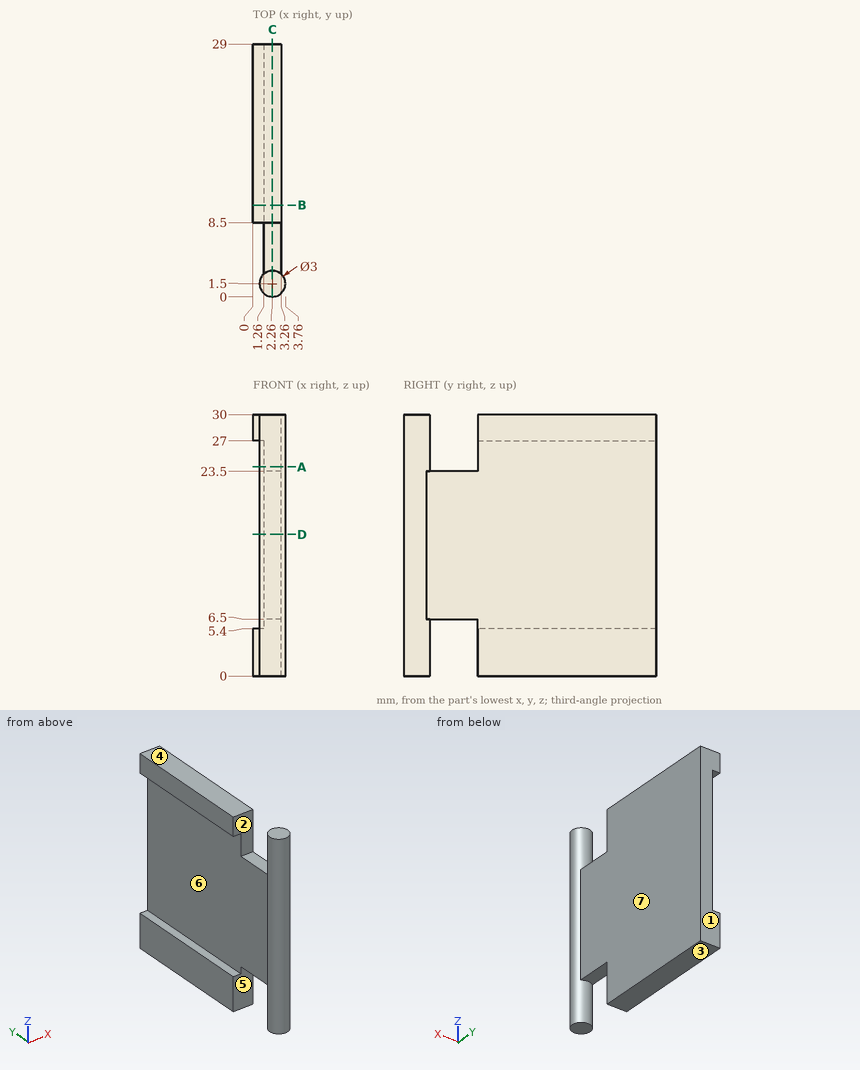
Check sheet for the drawn part. Datum: minimum x, y, z corner. Units: mm. A direction names the side the tool comes from. Round coordinates to 2 decimals unless told otherwise and drop trailing zeros. Order: outer loops, then holes, each group sorted by start corner. A loop starts at its lowest first (then second) coordinate and runs counter-clockwise, first axis right, second up. Notation, with made-up numbers: (25.5, 72.25) -> (70.5, 72.25) arc R26 ccw to (70.5, 103.25) -> close; hole circle Ø7 at (-24, -5). An arc over 180 degrees is marked (long way). Use CSV: the item, a comma, the result in double quotes.
(1) Cross-section at D-D (z = 16.25). Record the boundary of the cut face in (x, y).
Worked out:
outline,"(1.26, 2.62) arc R1.5 ccw (long way) to (3.26, 2.62) -> (3.26, 29) -> (1.26, 29) -> close"
(2) Draft check along Y on the marked faces 1, 2 and 3. Enter one of: pulls with the +Y half, pulls with the -Y half, needs draft (parallel to the pull), parting line crosses it, or undercut.
Worked out:
face 1,"pulls with the +Y half"
face 2,"undercut"
face 3,"needs draft"
(3) Cross-section at A-A (z = 24). Record the boundary of the cut face in (x, y), and give its area (3 significant figures).
Worked out:
outline,"circle Ø3 at (2.26, 1.5); (1.26, 8.5) -> (3.26, 8.5) -> (3.26, 29) -> (1.26, 29) -> close"
area,"48.1 mm²"
(4) Tool access check on the marked faces 4, 5, 6 and 7. Record the directions out of +Z, -Z, +X, -X, +Y, -Y that give a thin tool (end or side, any length) a straight path to the whole face; none if there is none.
Worked out:
face 4,"+Z, +X, -X, +Y, -Y"
face 5,"-Z, +X, -X"
face 6,"-X, +Y"
face 7,"+Z, -Z, +X, +Y"
(5) Cross-section at C-C (x = 2.26). Record the boundary of the cut face in (y, z).
Worked out:
outline,"(0, 0) -> (3, 0) -> (3, 6.5) -> (8.5, 6.5) -> (8.5, 0) -> (29, 0) -> (29, 30) -> (8.5, 30) -> (8.5, 23.5) -> (3, 23.5) -> (3, 30) -> (0, 30) -> close"
(6) Cross-section at B-B (y = 10.5). Record the boundary of the cut face in (x, z).
Worked out:
outline,"(0, 0) -> (3.26, 0) -> (3.26, 30) -> (0, 30) -> (0, 27) -> (1.26, 27) -> (1.26, 5.4) -> (0, 5.4) -> close"
(7) Depth check by flat-ended pin: pin 1 (0.6 mm diameter, centred on x = 2.5, y = 5.5, fed in from -Z); pin 2 (11 mm diameter, centred on y = 19.5, z = 16.5, fed in from -X); pin 3 (13 mm diameter, centred on y = 13.5, z = 11.5, fed in from +X). Enter the tip coordinate at first touch or a pass-through.
Worked out:
pin 1,"z = 6.5"
pin 2,"x = 1.26"
pin 3,"x = 3.26"
(8) Material ranges on line 1 along Z through (x, y) = (1.2, 21); line 2 along X through (y, z) = (18.75, 2.25); line 3 along X through (y, z) = (19.25, 9.5), recorded low to high. Write a range as from..to.
Worked out:
line 1,"0..5.4, 27..30"
line 2,"0..3.26"
line 3,"1.26..3.26"
